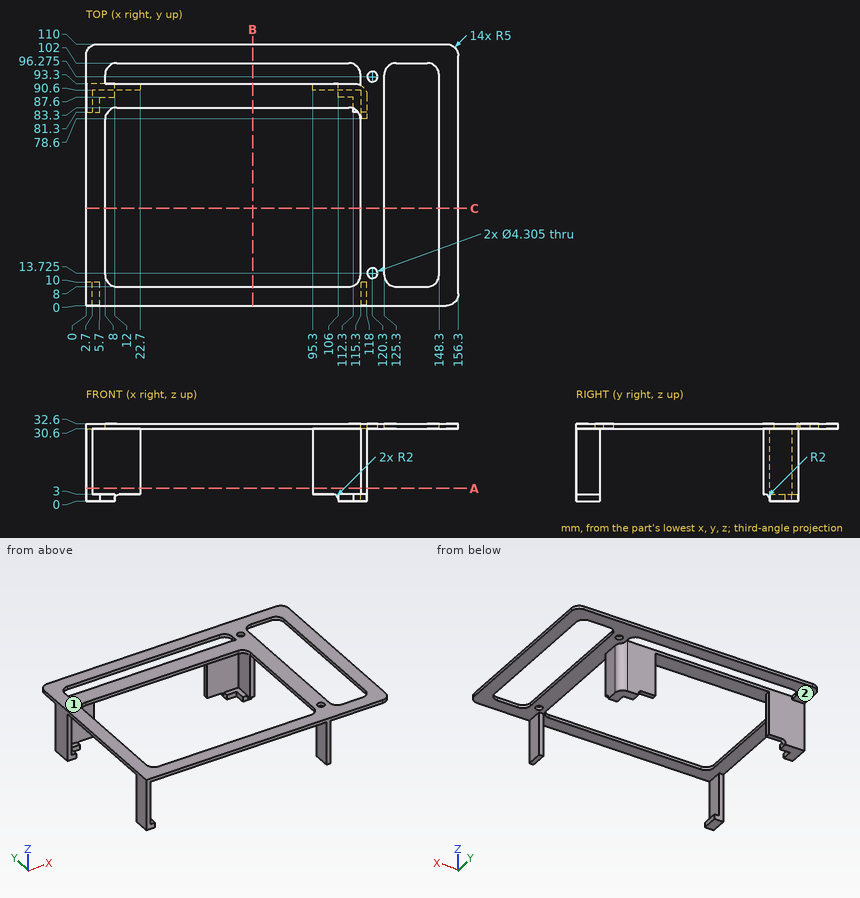
Design review of the part shown in the three views and the two pictorial views. Dimensions are in mm from the part's minimum x, y and z. Round coordinates to 2 decimals unless told otherwise and drop trailing zeros. Order: outer loops, then holes, each group sorted by start corner. A loop starts at its lowest first (then second) coordinate and runs counter-clockwise, first axis right, second up. Notation, with made-up numbers: (76.5, -37) -> (125.5, -37) arc R9 cw to (125.5, -32) -> close; hole circle Ø8 at (-11.5, -39). An arc over 180 degrees is marked (long way). Write item = value, one per line. Start each with the question number.
1) Insertion check: pin 1 (5 mm diameter, centred on y = 85, z = 15.5, fed in from +X); pin 2 (0.8 mm diameter, centred on x = 116.5, y = 79, fed in from -Z); pin 3 (2 mm diameter, centred on y = 91.5, z = 16, fed in from +X). Each pin has a flat end and moves straight along its axis. Give the tip position at first contact, or say it passes through.
2) Take a section at C-C on y = 41. State the section outline as (x, z) points.
3) Take a section at A-A on z = 5.5. State the section outline as (x, y) points.
4) The part is to be moulded in two halves that separate along X. For the marked faces 1 and 2, say which applies: +X half, -X half, draft (parallel to the pull), parting line (faces both ways), or undercut.
5) To check wall thickness, follow line 1 (Y direction, x = 120.3, z = 31.25); line 2 (X direction, y = 83.5, z = 22.5); line 3 (Z direction, x = 110, y = 85.5). State the ranges of each line that lie inside material, in increasing order. Write a range as from..to.
6) Take a section at B-B on x = 70. State the section outline as (y, z) points, plus the area to 3 significant figures.
Verdict:
q1.pin_1 = 118
q1.pin_2 = 3
q1.pin_3 = 117.49
q2.outline = (0, 30.6) -> (8, 30.6) -> (8, 32.6) -> (0, 32.6) -> close; (115.3, 30.6) -> (125.3, 30.6) -> (125.3, 32.6) -> (115.3, 32.6) -> close; (148.3, 30.6) -> (156.3, 30.6) -> (156.3, 32.6) -> (148.3, 32.6) -> close
q3.outline = (0, 0) -> (2.7, 0) -> (2.7, 10) -> (0, 10) -> close; (0, 81.3) -> (2.7, 81.3) -> (2.7, 90.6) -> (22.7, 90.6) -> (22.7, 93.3) -> (0, 93.3) -> close; (95.3, 90.6) -> (115.3, 90.6) -> (115.3, 78.6) -> (118, 78.6) -> (118, 88.3) arc R5 ccw to (113, 93.3) -> (95.3, 93.3) -> close; (115.3, 0) -> (118, 0) -> (118, 10) -> (115.3, 10) -> close
q4.face_1 = draft
q4.face_2 = undercut
q5.line_1 = 0..11.57, 15.88..94.12, 98.43..110
q5.line_2 = 0..2.7, 115.3..118
q5.line_3 = 30.6..32.6
q6.outline = (0, 30.6) -> (8, 30.6) -> (8, 32.6) -> (0, 32.6) -> close; (83.3, 30.6) -> (93.3, 30.6) -> (93.3, 32.6) -> (83.3, 32.6) -> close; (102, 30.6) -> (110, 30.6) -> (110, 32.6) -> (102, 32.6) -> close
q6.area = 52.0 mm2
